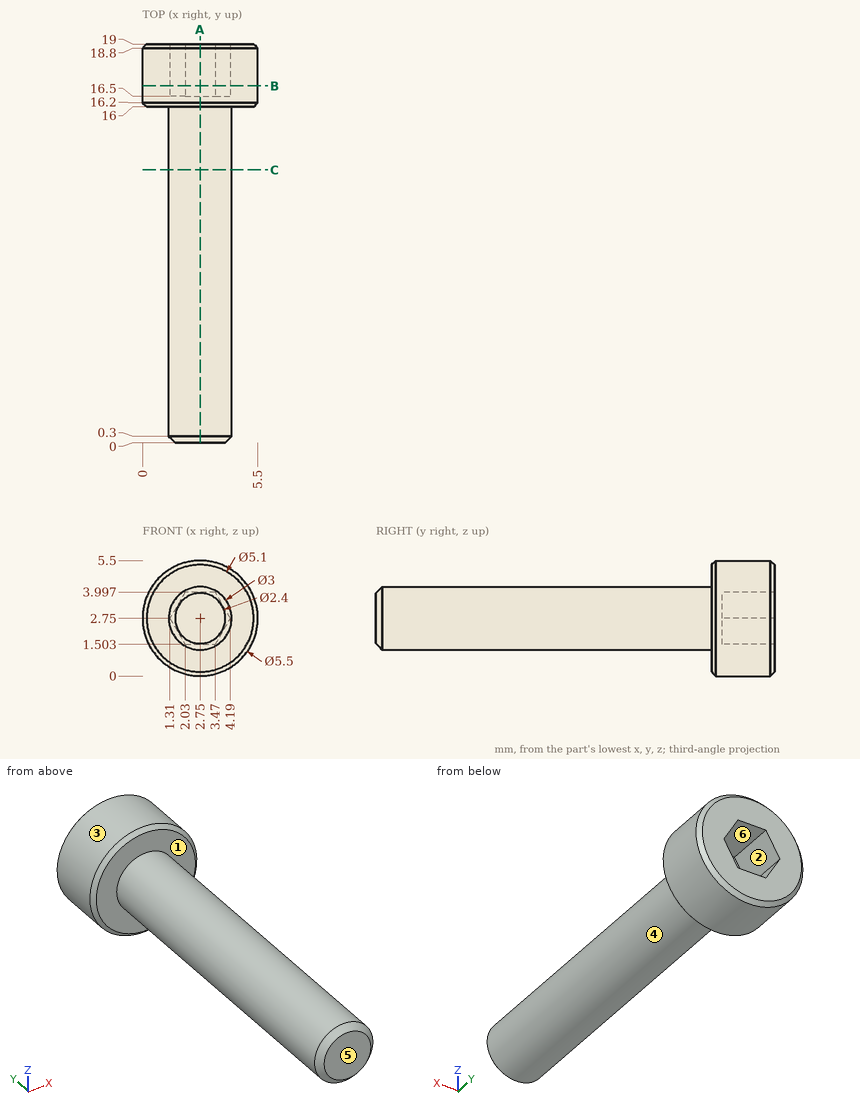
The figure shows three views and two pictorial views of one solid part (mm, origin at its lowest corner). Answer the questions. A direction names the side the tool comes from. Give positions to 0.01 mm unless a question says otherwise; leave off trailing zeros. Order: outer loops, then holes, each group sorted by start corner. A loop starts at its lowest first (then second) coordinate and runs counter-clockwise, first axis right, second up. Notation, with made-up numbers: (-35, 0) -> (-25, 0) arc R10 cw to (-25, 7) -> close; hole circle Ø2 at (70.5, 80.25). An arc over 180 degrees is marked (long way). Answer as a JSON object with one key per item and string values. Group by question number.
Item 1: Determine the mould class of the marked faces 1, 2 and 3 for opening direction Z: pulls with the +Z half, pulls with the -Z half, needs draft (parallel to the pull), parting line crosses it, or undercut.
Item 2: The part is cut by section C-C on y = 13. Write down the section's boundary in (x, z), and give its area (3 significant figures).
Item 3: A tool of negligible diameter and unlimited length cuts with its end or side. For the marked faces 4, 5 and 6, from which of +Z, -Z, +X, -X, +Y, -Y can it reach the whole face along a straight path? Write none if from no direction.
Item 4: Consider L1, parallel to Y at x = 2.45, z = 2.2; L2, parallel to Y at x = 3.5, z = 5.15; L3, parallel to X at y = 15, z = 2.65. Determine where each line is inside the solid, lowest interval first. Write a range as from..to.
Item 5: The part is cut by section B-B on y = 17. Write down the section's boundary in (x, z), and give its area (3 significant figures).
Item 6: The part is cut by section A-A on x = 2.75. Write down the section's boundary in (y, z).
Item 7: Flat-ended cylindrical pins translate along their axes: pin 1 (1 mm diameter, centred on x = 2.5, y = 7, fed in from +Z); pin 2 (3 mm diameter, centred on x = 3.5, y = 13.5, fed in from -Z). Find the tip coordinate at first contact, or state that the pin passes through.
Result set:
{
 "1": {"face 1": "needs draft", "face 2": "undercut", "face 3": "parting line crosses it"},
 "2": {"outline": "circle Ø3 at (2.75, 2.75)", "area": "7.07 mm²"},
 "3": {"face 4": "-Y", "face 5": "+Z, -Z, +X, -X, -Y", "face 6": "+Y"},
 "4": {"L1": "0..16.5", "L2": "16..19", "L3": "1.25..4.25"},
 "5": {"outline": "circle Ø5.5 at (2.75, 2.75); hole (1.31, 2.75) -> (2.03, 1.5) -> (3.47, 1.5) -> (4.19, 2.75) -> (3.47, 4) -> (2.03, 4) -> close", "area": "18.4 mm²"},
 "6": {"outline": "(0, 1.55) -> (0.3, 1.25) -> (16, 1.25) -> (16, 0.2) -> (16.2, 0) -> (18.8, 0) -> (19, 0.2) -> (19, 1.5) -> (16.5, 1.5) -> (16.5, 4) -> (19, 4) -> (19, 5.3) -> (18.8, 5.5) -> (16.2, 5.5) -> (16, 5.3) -> (16, 4.25) -> (0.3, 4.25) -> (0, 3.95) -> close"},
 "7": {"pin 1": "z = 4.25", "pin 2": "z = 1.25"}
}
